Read the model definition and answer for the solid it produces. Units are mm, in the model's axes. Face numbers are marked on the shaded views. A direction names the side the tool comes from. Round coordinates to 2 decimals unless told otherwise and drop trailing zeros. Write each loop counter-clockwise with the first axis right and the second up, starting at its lowest first coordinate (ties: lowest second). Pieces come first, ordered by that corner, then holes. Notation, with made-up numbers: (21.5, -32.5) -> (74.5, -32.5) arc R32 ccw to (74.5, 4.5) -> close; hole circle Ø3 at (58.25, 30). An arc over 180 degrees is marked (long way). Return JSON: item names as keys, results as strings.
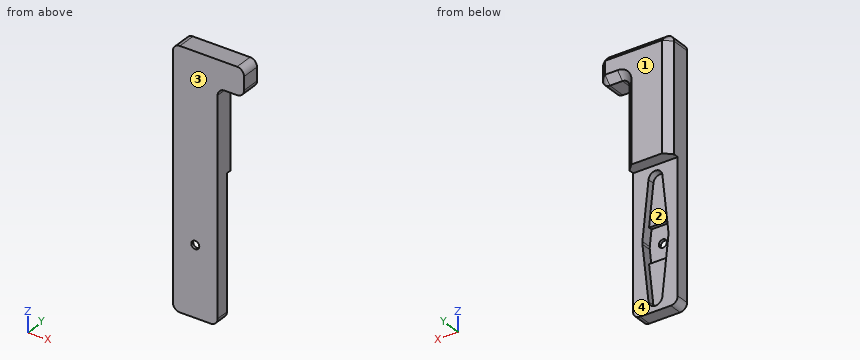
Autodesk Inventor part; units mm, degrees
ref_plane "YZ Plane" through (0, 0, 0) normal (1, 0, 0) x (0, 1, 0)
ref_plane "XZ Plane" through (0, 0, 0) normal (0, 1, 0) x (-1, 0, 0)
ref_plane "XY Plane" through (0, 0, 0) normal (0, 0, 1) x (1, 0, 0)
sketch "Sketch1" plane through (0, 0, 0) normal (0, 1, 0) x (-1, 0, 0)
  circle A0 centre (0, 0) radius 3.75
  circle A1 centre (0, 16.5) radius 2
  line L0 (0, 16.5) -> (0, 0) construction
  line L1 (1.9887, 16.7121) -> (3.7288, 0.3977)
  line L2 (-3.7288, 0.3977) -> (-1.9887, 16.7121)
  line L3 (0, 16.5) -> (0, 18.5) construction
  line L4 (0, 0) -> (3.75, 0) construction
  circle A2 centre (0, -16.5) radius 2
  line L5 (0, -16.5) -> (0, -18.5) construction
  line L6 (1.9887, -16.7121) -> (3.7288, -0.3977)
  line L7 (0, -16.5) -> (0, 0) construction
  line L8 (-3.7288, -0.3977) -> (-1.9887, -16.7121)
  line L9 (3.238, 5) -> (-3.238, 5)
  line L10 (-3.238, -5) -> (3.238, -5)
  line L11 (-6.4, -20) -> (6.4, -20)
  line L12 (6.4, -20) -> (6.4, 20)
  line L13 (6.4, 20) -> (-6.4, 20)
  line L14 (-6.4, 20) -> (-6.4, -20)
  line L15 (-6.4, -20) -> (6.4, 20) construction
  line L16 (6.4, -20) -> (-6.4, 20) construction
  line L17 (6.4, 53) -> (-14, 53)
  line L18 (-14, 53) -> (-14, 45.2)
  line L19 (-14, 45.2) -> (-6.4, 45.2)
  line L20 (-6.4, 45.2) -> (-6.4, 20)
  line L21 (6.4, 53) -> (6.4, 20)
  line L22 (0, 20) -> (0, 53) construction
  point P0 (-3.7288, -0.3977)
  point P1 (3.7288, -0.3977)
  dimension "d0" = 4
  dimension "d1" = 7.5
  dimension "d2" = 18.5
  dimension "d3" = 5
  dimension "d4" = 5
  dimension "d7" = 12.8
  dimension "d8" = 40
  dimension "d9" = 6.4
  dimension "d10" = 6.4
  dimension "d11" = 53
  dimension "d12" = 14
  dimension "d13" = 7.8
extrude "Extrusion1" add sketch "Sketch1" against normal blind 1.8 contours A0 | A0 L2 L9 L1 | L6 L10 L8 A0 | L9 L2 A1 L1 | L6 A2 L8 L10 | A1 | A2 | L14 L13 L12 L11 | L20 L19 L18 L17 L21 L13
extrude "Extrusion2" add sketch "Sketch1" along normal blind 2 contours L14 L13 L12 L11
hole "Hole2" at (0, 0, 0) direction (0, -1, 0) diameter 2.3 end through all
extrude "Extrusion3" cut sketch "Sketch1" against normal blind 1 contours A0 | A0 L2 L9 L1 | L6 L10 L8 A0
extrude "Extrusion4" add sketch "Sketch1" along normal blind 5.5 contours L20 L19 L18 L17 L21 L13
fillet "Fillet1" radius 2 6 edges at (6.4, 1.85, 45.2) (14, 1.85, 45.2) (14, 1.85, 53) (-6.4, 1.85, 53) (6.4, 0.1, -20) (-6.4, 0.1, -20)
chamfer "Chamfer1" distance 2 angle 45 8 edges at (6.4, 5.5, 31.6) (10.2, 5.5, 45.2) (13.4142, 5.5, 45.7858) (14, 5.5, 49.1) (13.4142, 5.5, 52.4142) (3.8, 5.5, 53) (-5.8142, 5.5, 52.4142) (-6.4, 5.5, 35.5)
equation "\"d7\" = 2 * d9"
equation "\"d10\" = d9"
properties part number "arm2_3DPrint"
Item 1: Section D-D (z = -2.5) is taken. Give the vertices of the cut face in (x, y).
Worked answers:
{"outline": "(-6.4, -1.8) -> (6.4, -1.8) -> (6.4, 2) -> (3.5, 2) -> (3.5, -1) -> (-3.5, -1) -> (-3.5, 2) -> (-6.4, 2) -> close"}
Item 2: For a pull along X with two mould halves and no side action, classify the marked faces 1 and 2 as released by +X, released by -X, zero draft, split by the parting line, or undercut.
Worked answers:
{"face 1": "zero draft", "face 2": "undercut"}
Item 3: Flat-ended cylindrical pins translate along their axes: pin 1 (4 mm diameter, centred on y = 1.5, z = 0, fed in from +X); pin 2 (6.5 mm diameter, centred on x = 2.5, z = -1.5, fed in from +Y); pin 3 (1.9 mm diameter, centred on x = -0.5, z = 11.5, fed in from +Y). Find the tip coordinate at first contact, or state that the pin passes through.
Worked answers:
{"pin 1": "stops at x = 6.4", "pin 2": "stops at y = 2", "pin 3": "stops at y = 0"}
Item 4: Section B-B (z = 22) is taken. Give the vertices of the cut face in (x, y).
Worked answers:
{"outline": "(-6.4, -1.8) -> (6.4, -1.8) -> (6.4, 3.5) -> (4.4, 5.5) -> (-4.4, 5.5) -> (-6.4, 3.5) -> close"}
Item 5: Straight lines are drawn through the part: L1, parallel to Z at x = 0, y = -1.4; L2, parallel to X at y = -1.45, z = 0; L3, parallel to Z at x = 10.25, y = 0.5. For each, find the intervals that lie inside material, in ascending order. Write a range as [from, to].
Worked answers:
{"L1": "z = [-20, -1.15], [1.15, 53]", "L2": "x = [-6.4, -1.15], [1.15, 6.4]", "L3": "z = [45.2, 53]"}
Item 6: A tool of negligible diameter and unlimited length cuts with its end or side. For the marked faces 3 and 4, from which of +Z, -Z, +X, -X, +Y, -Y can it reach the whole face along a straight path? Write none if from no direction.
Worked answers:
{"face 3": "+Z, -Z, +X, -X, -Y", "face 4": "-Z, +X, -X, +Y"}
Item 7: Section A-A (x = 0) is taken. Give the vertices of the cut face in (y, z).
Worked answers:
{"outline": "(-1.8, -20) -> (2, -20) -> (2, -18.5) -> (0, -18.5) -> (0, -5) -> (-1, -5) -> (-1, -1.15) -> (-1.8, -1.15) -> close; (-1.8, 1.15) -> (-1, 1.15) -> (-1, 5) -> (0, 5) -> (0, 18.5) -> (2, 18.5) -> (2, 20) -> (5.5, 20) -> (5.5, 51) -> (3.5, 53) -> (-1.8, 53) -> close"}
Item 8: Section C-C (y = 4.25) is taken. Give the vertices of the cut face in (x, z).
Worked answers:
{"outline": "(-5.65, 20) -> (5.65, 20) -> (5.65, 43.2) arc R2.75 cw to (8.4, 45.95) -> (12, 45.95) arc R1.25 ccw to (13.25, 47.2) -> (13.25, 51) arc R1.25 ccw to (12, 52.25) -> (-4.4, 52.25) arc R1.25 ccw to (-5.65, 51) -> close"}
